Source: CAD feature listing. Evaluate the final solid. Frame: model axes, mm. Face numbers are marked on the shaded views. A direction names the side the tool comes from. Round coordinates to 2 decimals unless told otherwise and drop trailing zeros. Loops run counter-clockwise (first coordinate to the right, second up) from the corner with the lowest first, then second, coordinate; pieces in that order, holes last. Notation, with made-up numbers: (65.25, 70) - (98.25, 70) arc R21 cw to (98.25, 103) - close; hole circle Ø7 at (11, 63). An arc over 180 degrees is marked (long way). Write item = value, one per line. Start each with the question number.
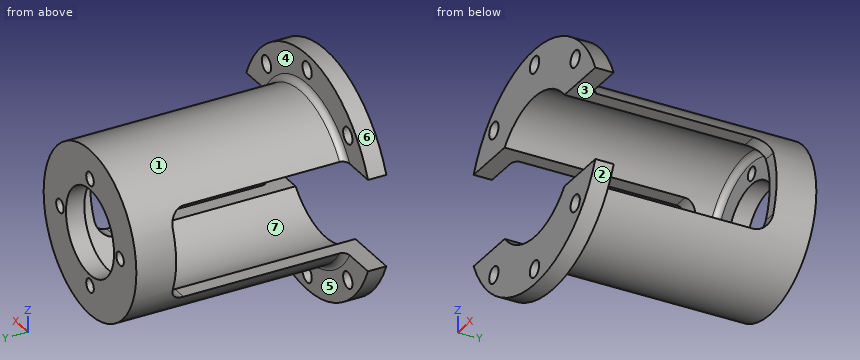
from build123d import *

# Parameters (mm, degrees)
SKETCH1_R               = 27
SKETCH1_R_2             = 23
BOSS_EXTRUDE1_DEPTH     = 77
BOSS_EXTRUDE2_START     = -6
SKETCH2_R               = 27
BOSS_EXTRUDE2_DEPTH     = 6
SKETCH3_R               = 38.5
SKETCH3_R_2             = 23
BOSS_EXTRUDE3_DEPTH     = 6
SKETCH4_R               = 14
CUT_EXTRUDE1_DEPTH      = 95.305355097
CUT_EXTRUDE2_DEPTH      = 95.305355097
CUT_EXTRUDE2_DEPTH_BACK = 95.305355097
FILLET1_R               = 2
SKETCH7_R               = 2.7
CUT_EXTRUDE3_DEPTH      = 89.207142689
CIRPATTERN1_COUNT       = 8
SKETCH8_R               = 2.2
CUT_EXTRUDE4_DEPTH      = 94.104779805
CIRPATTERN2_COUNT       = 4


with BuildPart() as part:
    # Sketch1 → Boss-Extrude1 (new body)
    with BuildSketch(Plane(origin=(0, 0, 0), x_dir=(1, 0, 0), z_dir=(0, 1, 0))):
        with Locations(Location((0, 0, 0), (0, 0, 270))):
            Circle(SKETCH1_R)
        with Locations(Location((0, 0, 0), (0, 0, 270))):
            Circle(SKETCH1_R_2, mode=Mode.SUBTRACT)
    extrude(amount=BOSS_EXTRUDE1_DEPTH)

    # Sketch2 → Boss-Extrude2 (add)
    with BuildSketch(Plane(origin=(0, 77, 0), x_dir=(1, 0, 0), z_dir=(0, 1, 0)).offset(BOSS_EXTRUDE2_START)):
        with Locations(Location((0, 0, 0), (0, 0, 270))):
            Circle(SKETCH2_R)
    extrude(amount=BOSS_EXTRUDE2_DEPTH)

    # Sketch3 → Boss-Extrude3 (add)
    with BuildSketch(Plane.XZ):
        with Locations(Location((0, 0, 0), (0, 0, 270))):
            Circle(SKETCH3_R)
        with Locations(Location((0, 0, 0), (0, 0, 90))):
            Circle(SKETCH3_R_2, mode=Mode.SUBTRACT)
    extrude(amount=-BOSS_EXTRUDE3_DEPTH)

    # Sketch4 → Cut-Extrude1 (cut, through all)
    with BuildSketch(Plane(origin=(0, 77, 0), x_dir=(1, 0, 0), z_dir=(0, 1, 0))):
        with Locations(Location((0, 0, 0), (0, 0, 270))):
            Circle(SKETCH4_R)
    extrude(amount=-CUT_EXTRUDE1_DEPTH, mode=Mode.SUBTRACT)

    # Sketch5 → Cut-Extrude2 (cut, two sides: drawn at the far end of the back side and taken through both)
    with BuildSketch(Plane(origin=(0, 0, 0), x_dir=(0, 0, -1), z_dir=(1, 0, 0)).offset(-CUT_EXTRUDE2_DEPTH_BACK)):
        with BuildLine():
            Line((-15, 0), (-15, 59))
            ThreePointArc((-15, 59), (-13.535533906, 62.535533906), (-10, 64))
            Line((-10, 64), (10, 64))
            ThreePointArc((10, 64), (13.535533906, 62.535533906), (15, 59))
            Line((15, 59), (15, 0))
            Line((15, 0), (-15, 0))
        make_face()
    extrude(amount=CUT_EXTRUDE2_DEPTH + CUT_EXTRUDE2_DEPTH_BACK, mode=Mode.SUBTRACT)

    # Fillet1
    fillet1_edges = [part.edges().sort_by_distance(p)[0] for p in [
        (0, 71, -23),
        (12.727922061, 6, 23.8117618),
        (0, 6, -27),
    ]]
    fillet(fillet1_edges, radius=FILLET1_R)

    # Sketch7 → Cut-Extrude3 (cut, through all)
    with BuildSketch(Plane(origin=(0, 6, 0), x_dir=(1, 0, 0), z_dir=(0, 1, 0))):
        with Locations(Location((0, 33.5, 0), (0, 0, 270))):
            Circle(SKETCH7_R)
    cut_extrude3 = extrude(amount=-CUT_EXTRUDE3_DEPTH, mode=Mode.SUBTRACT)

    # CirPattern1: Cut-Extrude3 ×8 about axis, 2 skipped
    cirpattern1_axis = Axis((0, 0, 0), (0, 1, 0))
    add([cut_extrude3.rotate(cirpattern1_axis, i * 360 / CIRPATTERN1_COUNT) for i in range(1, CIRPATTERN1_COUNT) if i not in (2, 6)], mode=Mode.SUBTRACT)

    # Sketch8 → Cut-Extrude4 (cut, through all)
    with BuildSketch(Plane(origin=(0, 77, 0), x_dir=(1, 0, 0), z_dir=(0, 1, 0))):
        with Locations(Location((0, 17.5, 0), (0, 0, 270))):
            Circle(SKETCH8_R)
    cut_extrude4 = extrude(amount=-CUT_EXTRUDE4_DEPTH, mode=Mode.SUBTRACT)

    # CirPattern2: Cut-Extrude4 ×4 about axis
    cirpattern2_axis = Axis((0, 0, 0), (0, 1, 0))
    for i in range(1, CIRPATTERN2_COUNT):
        add(cut_extrude4.rotate(cirpattern2_axis, i * 360 / CIRPATTERN2_COUNT), mode=Mode.SUBTRACT)


solid = part.part
(1) Cut plane D-D (z = -33.5). Output: boundary loops of the cut face in (x, y).
(2) Mould query, pull axis Z, two halves, no side actions, for the marked faces 1, 2, 3 and 4. Classes: +Z half, -Z half, draft (parallel to the pull), parting line (faces both ways), or undercut.
(3) Pin query (flat end, axial travel): P1, Ø1, axis at x = -3.5, y = 41.5, coming from the -Z side; P2, Ø7, axis at x = 17.5, z = 0, coming from the -Y side; P3, Ø1, axis at x = 22, y = 31, coming from the +Z side; P4, Ø8.5, axis at x = 0, z = 33.5, coming from the -Y side. Return the tip coordinate at first contact, or that it passes through.
(4) Access query for the marked faces 5, 6 and 7. Directions: +Z, -Z, +X, -X, +Y, -Y. A direction counts if a zero-diameter tool reaches every point of the face in a straight line with its end or side. Return the directions, or none.
(5) Cut plane A-A (z = 0). Output: boundary loops of the cut face in (x, y).
(6) Material intervals for line 1 along Y through (x, z) = (-14.5, 15); line 2 along X through (y, z) = (3.3, 33.5); line 3 along Z through (x, y) = (8, 10), sorted ascending. Write a range as from..to.
(7) Cut plane B-B (y = 50). Output: boundary loops of the cut face in (x, z), and give its area (3 significant figures).
(8) Cut plane C-C (x = 0). State how many separate pieces and enclosed holes the cut face has, and give its area (3 significant figures).
Solution:
q1.outline = (-18.97, 0) - (-2.7, 0) - (-2.7, 6) - (-18.97, 6) - close; (2.7, 0) - (18.97, 0) - (18.97, 6) - (2.7, 6) - close
q2.face_1 = parting line
q2.face_2 = -Z half
q2.face_3 = undercut
q2.face_4 = draft
q3.P1 = -26.83
q3.P2 = 71
q3.P3 = 16.33
q3.P4 = 0
q4.face_5 = -Z, +Y
q4.face_6 = +Z, +Y, -Y
q4.face_7 = -Y
q5.outline = (-27, 64) - (-23, 64) - (-23, 69) arc R2 cw to (-21, 71) - (-19.7, 71) - (-19.7, 77) - (-27, 77) - close; (-15.3, 71) - (-14, 71) - (-14, 77) - (-15.3, 77) - close; (14, 71) - (15.3, 71) - (15.3, 77) - (14, 77) - close; (19.7, 71) - (21, 71) arc R2 cw to (23, 69) - (23, 64) - (27, 64) - (27, 77) - (19.7, 77) - close
q6.line_1 = 71..77
q6.line_2 = -18.97..-2.7, 2.7..18.97
q6.line_3 = -25.79..-21.56, 21.56..25.79
q7.outline = (-22.45, -15) arc R27 ccw to (22.45, -15) - (17.44, -15) arc R23 cw to (-17.44, -15) - close; (-22.45, 15) - (-17.44, 15) arc R23 cw to (17.44, 15) - (22.45, 15) arc R27 ccw to start
q7.area = 371 mm^2
q8.separate_pieces = 6
q8.enclosed_holes = 0
q8.area = 748 mm^2
